Check sheet for the modelled part. Datum: model origin and axes. Units: mm. Face numbers are marked on the shaded views. A direction names the side the tool comes from. Give positions to 0.01 mm unless a question says otherwise; leave off trailing zeros. Write each loop counter-clockwise with the first axis right and the second up, starting at its lowest first coordinate (ties: lowest second). Pieces come first, ordered by that corner, then holes. Notation, with made-up numbers: (71, -29.5) -> (79, -29.5) arc R11 cw to (79, -20.5) -> close; hole circle Ø4 at (69.25, -11.75). An arc over 180 degrees is marked (long way). Use a Markdown table: item, result. Add a question column.
1. Cross-section at A-A (x = -4). Enter the section's corners in (y, z).
2. Cross-section at B-B (y = -23). Enter the section's corners in (x, z).
3. Release check for a two-part mould opening along X. For the marked faces 1, 2 and 3 record: released by +X, released by -X, zero draft, split by the parting line, or undercut.
4. Cross-section at C-C (z = 7). Enter the section's corners in (x, y), then the cut area to 3 significant figures.
5. Scan lines: probe 1 along Y at (x, z) = (0, 58); probe 2 along Y at (x, z) = (-8, 58.35); probe 3 along Z at (x, y) = (-6, -7). Record each from-to range of solid material in increasing order. Write a range as [from, to].
6. Gauge pin test, flat ends, axial feed: P1, Ø2.5, axis at x = 0, y = -8, coming from the -Z side; P2, Ø5, axis at y = 3, z = 9.5, coming from the -X side; P3, Ø12, axis at x = -50.5, z = 23.5, coming from the +Y side; P4, Ø12, axis at x = 39, z = 15.5, coming from the -Y side. Record the tip position at first contact, or that the pin passes through.
7. Set-up check for the marked faces 4 and 5: record each of +Z, -Z, +X, -X, +Y, -Y from which the full face is reachable in a straight line by a thin tool's end or side.
8. Cross-section at D-D (y = 15). Enter the section's corners in (x, z).
from build123d import *

# Parameters (mm, degrees)
F0_W          = 134
F0_H          = 80
F1_DEPTH      = 4
F2_W          = 128
F2_H          = 74
F2_W_2        = 122
F2_H_2        = 68
F3_DEPTH      = 2
F3_DEPTH_BACK = 4
F5_DEPTH      = 17.5
F6_R          = 1.2120191714
F6_R_2        = 1
F9_DEPTH      = 25
F7_R          = 1.4559122593
F7_R_2        = 1
F10_DEPTH     = 25
F8_R          = 1.2120191714
F8_R_2        = 1
F11_DEPTH     = 25
F12_R         = 15


with BuildPart() as f1:
    # F0 (on Top) → F1 (new body)
    with BuildSketch(Plane.XY):
        Rectangle(F0_W, F0_H)
    extrude(amount=F1_DEPTH)

    # F2 (on face) → F3 (cut, two sides)
    with BuildSketch(Plane(origin=(0, 0, 0), x_dir=(1, 0, 0), z_dir=(0, 0, -1))) as f3_sk:
        Rectangle(F2_W, F2_H)
        Rectangle(F2_W_2, F2_H_2, mode=Mode.SUBTRACT)
        Rectangle(F2_W_2, F2_H_2)
    extrude(amount=F3_DEPTH, mode=Mode.SUBTRACT)
    extrude(f3_sk.sketch, amount=-F3_DEPTH_BACK, mode=Mode.SUBTRACT)

    # F4 (on Front) → F5 (join, symmetric)
    with BuildSketch(Plane.XZ):
        Polygon((-27.5, 59), (-65.2364429114, 18.9879908478), (-67, 4), (-64, 4), (-62.3966282188, 17.6266195959), (-26.205621828, 56), (26.166218832, 56), (61.6182726396, 16.71034506), (64, 4), (67, 4), (64.3454915045, 18.1660710219), (27.5, 59), align=None)
    extrude(amount=F5_DEPTH, both=True)

    # F6 (on face) → F9 (cut)
    with BuildSketch(Plane.XY.offset(59)):
        Circle(F6_R)
        with Locations((-8, 0)):
            Circle(F6_R_2)
        with Locations((0, -8)):
            Circle(F6_R_2)
        with Locations((8, 0)):
            Circle(F6_R_2)
        with Locations((0, 8)):
            Circle(F6_R_2)
    extrude(amount=-F9_DEPTH, mode=Mode.SUBTRACT)

    # F7 (on face) → F10 (cut)
    with BuildSketch(Plane(origin=(-44.0036916199, 0, 41.501110089), x_dir=(0, -1, 0), z_dir=(-0.7274910755, 0, 0.6861171438))):
        with Locations((0, -4.9021602608)):
            Circle(F7_R)
        with Locations((-7.9994338844, -4.8069892056)):
            Circle(F7_R_2)
        with Locations((-0.0951710552, -12.9015941452)):
            Circle(F7_R_2)
        with Locations((7.9994338844, -4.997331316)):
            Circle(F7_R_2)
        with Locations((0.0951710552, 3.0972736235)):
            Circle(F7_R_2)
    extrude(amount=-F10_DEPTH, mode=Mode.SUBTRACT)

    # F8 (on face) → F11 (cut)
    with BuildSketch(Plane(origin=(44.5031382137, 0, 40.1563122143), x_dir=(0, 1, 0), z_dir=(0.7424350723, 0, 0.6699180274))):
        with Locations((0, -2.1190764849)):
            Circle(F8_R)
        with Locations((-8, -2.1190764849)):
            Circle(F8_R_2)
        with Locations((0, -10.1190764849)):
            Circle(F8_R_2)
        with Locations((8, -2.1190764849)):
            Circle(F8_R_2)
        with Locations((0, 5.8809235151)):
            Circle(F8_R_2)
    extrude(amount=-F11_DEPTH, mode=Mode.SUBTRACT)

    # F12
    f12_edges = [f1.edges().sort_by_distance(p)[0] for p in [
        (26.166219, 0, 56),
        (-26.205622, 0, 56),
        (61.618273, 0, 16.710345),
        (-62.396628, 0, 17.62662),
    ]]
    fillet(f12_edges, radius=F12_R)


solid = f1.part
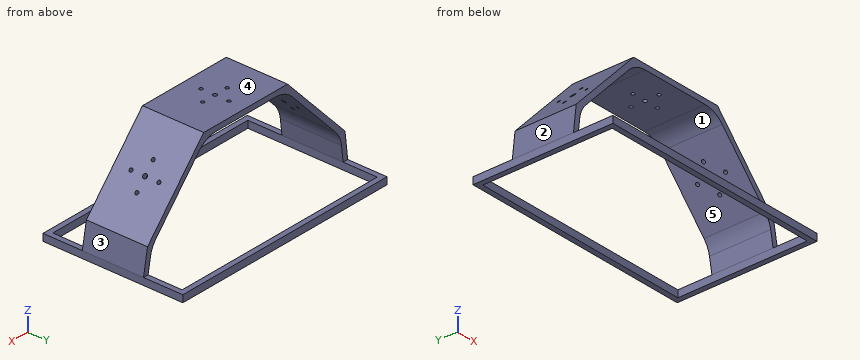
Worked answers:
| question | item | result |
|---|---|---|
| 1 | outline | (-40, 0) -> (-37, 0) -> (-37, 4) -> (-40, 4) -> close; (-17.5, 56) -> (17.5, 56) -> (17.5, 59) -> (-17.5, 59) -> close; (37, 0) -> (40, 0) -> (40, 4) -> (37, 4) -> close |
| 2 | outline | (-67, 0) -> (-64, 0) -> (-64, 4) -> (-67, 4) -> close; (64, 0) -> (67, 0) -> (67, 4) -> (64, 4) -> close |
| 3 | face 1 | undercut |
| 3 | face 2 | released by -X |
| 3 | face 3 | released by +X |
| 4 | outline | (-66.65, -17.5) -> (-63.65, -17.5) -> (-63.65, 17.5) -> (-66.65, 17.5) -> close; (63.44, -17.5) -> (66.44, -17.5) -> (66.44, 17.5) -> (63.44, 17.5) -> close |
| 4 | area | 210 mm² |
| 5 | probe 1 | y = [-17.5, -9], [-7, -1.21], [1.21, 7], [9, 17.5] |
| 5 | probe 2 | y = [-17.5, -1], [1, 17.5] |
| 5 | probe 3 | z = [56, 59] |
| 6 | P1 | stops at z = 56 |
| 6 | P2 | stops at x = -66.65 |
| 6 | P3 | stops at y = 17.5 |
| 6 | P4 | passes through |
| 7 | face 4 | +Z, +X, -X, +Y, -Y |
| 7 | face 5 | -Z, +Y, -Y |
| 8 | outline | (-67, 0) -> (-64, 0) -> (-64, 4) -> (-62.98, 12.7) arc R15 cw to (-58.99, 21.24) -> (-30.65, 51.29) arc R15 cw to (-19.73, 56) -> (19.5, 56) arc R15 cw to (30.63, 51.05) -> (58.79, 19.85) arc R15 cw to (62.4, 12.56) -> (64, 4) -> (64, 0) -> (67, 0) -> (67, 4) -> (64.35, 18.17) -> (27.5, 59) -> (-27.5, 59) -> (-65.24, 18.99) -> (-67, 4) -> close |
